For this review, take the finished solid that the model builds, in its own axes (mm). A direction names the side the tool comes from. Coordinates: 2 decimals unless noted, no trailing zeros. Write each loop counter-clockwise with the first axis right and the second up, starting at its lowest first coordinate (ties: lowest second). Pieces come first, ordered by that corner, then holes. Notation, with made-up numbers: (74.25, 65) - (98.25, 65) arc R20 ccw to (98.25, 96) - close; hole circle Ø1 at (-23, -2.5). An arc over 180 degrees is marked (long way). Use one line per item in the form item = value. Start each with the question number.
1) Tool access review of faces 4 (the flat face through (3, 69.07, -69)), 5 (the flat face through (3, 2, 0)), 6 (the flat face through (3, 3, -140)): name each direction out of +Z, -Z, +X, -X, +Y, -Y from which nothing blocks a thin tool from reaching the whole face with its end or side.
2) We need section A-A (y = 43). Give the boundary of the cut face in (x, z), plus the area to 3 significant figures.
3) Mouldability with a two-part tool opening along Z and no side actions: class faces 1 (the flat face through (2.958, 59.855, 7.922)), 2 (the flat face through (2.96, 60.11, -147.62)), 3 (the cylindrical face through (2.958, 67.334, -4.958)) as pulls with the +Z half, pulls with the -Z half, needs draft (parallel to the pull), parting line crosses it, or undercut.
4) For L1, parallel to X at y = 7, z = -10; L2, parallel to Y at x = 2.1, z = -3; L3, parallel to Y at x = 4.1, z = -155, list the stretches that pass through material, from the lowest coordinate up. Write a range as from..to.
5) Insertion check: P1, Ø1, axis at y = 46, z = -16.5, coming from the -X side; P2, Ø1.1, axis at x = 3, y = 0.5, coming from the -Z side. Each pin has a flat end and moves straight along its axis. Give the tip position at first contact, or say it passes through.
6) We need section B-B (z = -90.5). Give the boundary of the cut face in (x, y).
```python
from build123d import *

# Parameters (mm, degrees)
SKETCH1_R                   = 1.5
BOSS_EXTRUDE1_DEPTH         = 6
TAP_DRILL_FOR_M3_TAP1_D     = 2.5
TAP_DRILL_FOR_M3_TAP1_DEPTH = 10
TAP_DRILL_FOR_M3_TAP1_TIP   = 0.751075774


with BuildPart() as part:
    # Sketch1 → Boss-Extrude1 (new body)
    with BuildSketch(Plane(origin=(0, 0, 0), x_dir=(0, 0, -1), z_dir=(1, 0, 0))):
        with BuildLine():
            Line((0, 0), (0, 5))
            Line((0, 5), (-18.599926487, 50.895524881))
            Line((-18.599926487, 50.895524881), (3.059200375, 69.069690242))
            Line((3.059200375, 69.069690242), (136.940799625, 69.069690242))
            Line((136.940799625, 69.069690242), (158.599926487, 50.895524881))
            Line((158.599926487, 50.895524881), (140, 5))
            Line((140, 5), (140, 0))
            Line((140, 0), (120, 0))
            Line((120, 0), (120, 1))
            ThreePointArc((120, 1), (119.627466942, 2.162476387), (118.648648649, 2.891891892))
            ThreePointArc((118.648648649, 2.891891892), (70, 11), (21.351351351, 2.891891892))
            ThreePointArc((21.351351351, 2.891891892), (20.372533058, 2.162476387), (20, 1))
            Line((20, 1), (20, 0))
            Line((20, 0), (0, 0))
        make_face()
        with Locations((-15, 50)):
            Circle(SKETCH1_R, mode=Mode.SUBTRACT)
        with Locations((155, 50)):
            Circle(SKETCH1_R, mode=Mode.SUBTRACT)
        with Locations((4.151111078, 66.069690242)):
            Circle(SKETCH1_R, mode=Mode.SUBTRACT)
        with Locations((135.848888922, 66.069690242)):
            Circle(SKETCH1_R, mode=Mode.SUBTRACT)
    extrude(amount=BOSS_EXTRUDE1_DEPTH)

    # Tap Drill for M3 Tap1
    with Locations(Plane(origin=(0, 0, 0), x_dir=(-1, 0, 0), z_dir=(0, -1, 0))):
        with Locations((-3, 10), (-3, 130)):
            Hole(TAP_DRILL_FOR_M3_TAP1_D / 2, depth=TAP_DRILL_FOR_M3_TAP1_DEPTH)
            with Locations((0, 0, -(TAP_DRILL_FOR_M3_TAP1_DEPTH + TAP_DRILL_FOR_M3_TAP1_TIP / 2))):  # 118° drill point
                Cone(0, TAP_DRILL_FOR_M3_TAP1_D / 2, TAP_DRILL_FOR_M3_TAP1_TIP, mode=Mode.SUBTRACT)


solid = part.part
```
Determined:
q1.face_4 = +Z, -Z, +X, -X, +Y
q1.face_5 = +Z, +X, -X, -Y
q1.face_6 = -Z, +X, -X, -Y
q2.outline = (0, -155.4) - (6, -155.4) - (6, 15.4) - (0, 15.4) - close
q2.area = 1,020 mm²
q3.face_1 = pulls with the +Z half
q3.face_2 = pulls with the -Z half
q3.face_3 = undercut
q4.L1 = 0..1.75, 4.25..6
q4.L2 = 0..65.11, 67.03..69.02
q4.L3 = 42.01..48.5, 51.5..53.92
q5.P1 = 0
q5.P2 = -140
q6.outline = (0, 9.59) - (6, 9.59) - (6, 69.07) - (0, 69.07) - close
